Autodesk Inventor part; units mm, degrees
ref_plane "YZ Plane" through (0, 0, 0) normal (1, 0, 0) x (0, 1, 0)
ref_plane "XZ Plane" through (0, 0, 0) normal (0, 1, 0) x (-1, 0, 0)
ref_plane "XY Plane" through (0, 0, 0) normal (0, 0, 1) x (1, 0, 0)
sketch "Sketch1" plane through (0, 0, 0) normal (0, 1, 0) x (-1, 0, 0)
  line L0 (76.2, 76.2) -> (-76.2, 76.2)
  line L1 (-76.2, 76.2) -> (-76.2, -76.2)
  line L2 (-76.2, -76.2) -> (76.2, -76.2)
  line L3 (76.2, -76.2) -> (76.2, 76.2)
  point P0 (0, 0)
  dimension "d0" = 152.4
  dimension "d1" = 152.4
  dimension "d2" = 76.2
  dimension "d3" = 76.2
extrude "Extrusion1" add sketch "Sketch1" along normal blind 12.7
sketch "Sketch4" plane through (0, 12.7, 0) normal (0, 1, 0) x (1, 0, 0)
  circle A0 centre (69.85, 69.85) radius 3.175
  circle A1 centre (69.85, -69.85) radius 3.175
  circle A2 centre (-67.31, -52.07) radius 3.175
  line L0 (76.2, 76.2) -> (-76.2, 76.2)
  line L1 (76.2, -76.2) -> (76.2, 76.2)
  line L2 (-76.2, -76.2) -> (76.2, -76.2)
  line L3 (-76.2, 76.2) -> (-76.2, -76.2)
  circle A3 centre (-67.31, 52.07) radius 3.175
  point P0 (0, 0)
  dimension "d20" = 6.35
  dimension "d21" = 6.35
  dimension "d22" = 6.35
  dimension "d23" = 6.35
  dimension "d24" = 6.35
  dimension "d25" = 6.35
  dimension "d26" = 6.35
  dimension "d27" = 24.13
  dimension "d28" = 8.89
  dimension "d32" = 6.35
  dimension "d33" = 24.13
  dimension "d34" = 8.89
extrude "Extrusion6" [suppressed]
fillet "Fillet1" [suppressed]
sketch "Sketch7" plane through (0, 12.7, 0) normal (0, 1, 0) x (1, 0, 0)
  arc A0 (-76.2, -19.8745) -> (-11.9351, -76.2) centre (52.3545, 61.976) ccw
  line L0 (76.2, 76.2) -> (-76.2, 76.2)
  line L1 (76.2, -76.2) -> (76.2, 76.2)
  line L2 (-76.2, 76.2) -> (-76.2, -76.2)
  line L3 (-76.2, -76.2) -> (76.2, -76.2)
  line L4 (-76.2, 76.2) -> (-76.2, -76.2)
  arc A1 (-11.9351, -76.2) -> (-76.2, -19.8745) centre (52.3545, 61.976) ccw
  point P0 (0, 0)
  point P1 (76.2, -60.325)
  point P2 (73.025, -60.325)
  point P3 (73.025, 63.5)
  point P4 (73.025, 60.325)
  point P5 (-73.025, 63.5)
  point P6 (76.2, 60.325)
  point P7 (73.025, -63.5)
  point P8 (-76.2, 60.325)
  point P9 (-74.6455, -22.2663)
  dimension "d46" = 304.8
  dimension "d47" = 14.224
  dimension "d48" = 23.8455
sketch "Sketch8" plane through (0, 12.7, 0) normal (0, 1, 0) x (1, 0, 0)
  circle A0 centre (-38.0726, -33.782) radius 1.4224
  circle A1 centre (-44.8036, -27.051) radius 1.4224
  circle A2 centre (-51.5346, -33.782) radius 1.4224
  circle A3 centre (-51.5346, 67.818) radius 1.4224
  circle A4 centre (-44.8036, 61.087) radius 1.4224
  circle A5 centre (-38.0726, 67.818) radius 1.4224
  circle A6 centre (-53.876, 3.1912) radius 1.4224
  circle A7 centre (-53.876, 3.1912) radius 1.4224
  circle A8 centre (-44.856, 3.1912) radius 1.4224
  line L0 (-40.346, 0.6734) -> (-58.386, 0.6734)
  line L1 (-40.346, 5.7089) -> (-40.346, 0.6734)
  line L2 (-40.346, 5.7089) -> (-58.386, 5.7089)
  line L3 (-58.386, 0.6734) -> (-58.386, 5.7089)
  circle A9 centre (-53.876, 31.1756) radius 1.4224
  circle A10 centre (-44.856, 31.1756) radius 1.4224
  line L4 (-40.346, 28.6579) -> (-58.386, 28.6579)
  line L5 (-40.346, 33.6934) -> (-40.346, 28.6579)
  line L6 (-40.346, 33.6934) -> (-58.386, 33.6934)
  line L7 (-58.386, 28.6579) -> (-58.386, 33.6934)
  circle A11 centre (2.54, -39.6875) radius 3.175 construction
  circle A12 centre (2.54, 12.7127) radius 3.175 construction
  circle A13 centre (2.54, 65.1129) radius 3.175 construction
  circle A14 centre (68.58, 65.1129) radius 3.175 construction
  circle A15 centre (68.58, 12.7127) radius 3.175 construction
  circle A16 centre (68.58, -39.6875) radius 3.175 construction
extrude "Extrusion9" cut sketch "Sketch8" against normal through all contours A0 | A1 | A2 | A3 | A4 | A5 | A6 | A8 | A9 | A10
extrude "Extrusion11" cut sketch "Sketch7" against normal through all contours A0 L3 L2
sketch "Sketch10" plane through (0, 12.7, 0) normal (0, 1, 0) x (1, 0, 0)
  circle A0 centre (68.961, 72.39) radius 1.4732
  arc A1 (-76.2, -19.8745) -> (-11.9351, -76.2) centre (52.3545, 61.976) ccw
  line L0 (-11.9351, -76.2) -> (76.2, -76.2)
  line L1 (76.2, -76.2) -> (76.2, 76.2)
  line L2 (76.2, 76.2) -> (-76.2, 76.2)
  line L3 (-76.2, 76.2) -> (-76.2, -19.8745)
  circle A2 centre (-53.876, 31.1756) radius 1.4224
  circle A3 centre (-53.876, 3.1912) radius 1.4224
  circle A4 centre (-44.8036, 61.087) radius 1.4224
  circle A5 centre (-51.5346, -33.782) radius 1.4224
  circle A6 centre (-38.0726, -33.782) radius 1.4224
  circle A7 centre (-44.8036, -27.051) radius 1.4224
  circle A8 centre (-51.5346, 67.818) radius 1.4224
  circle A9 centre (-38.0726, 67.818) radius 1.4224
  circle A10 centre (-44.856, 3.1912) radius 1.4224
  circle A11 centre (-44.856, 31.1756) radius 1.4224
  circle A12 centre (40.005, 72.39) radius 1.4732
  circle A13 centre (54.483, 72.39) radius 1.4732
  circle A14 centre (25.527, 72.39) radius 1.4732
  circle A15 centre (11.049, 72.39) radius 1.4732
  circle A16 centre (68.961, -68.58) radius 1.4732
  circle A17 centre (54.483, -68.58) radius 1.4732
  circle A18 centre (40.005, -68.58) radius 1.4732
  circle A19 centre (25.527, -68.58) radius 1.4732
  circle A20 centre (11.049, -68.58) radius 1.4732
  point P0 (0, 0)
extrude "Extrusion13" cut sketch "Sketch10" against normal through all contours A0 | A12 | A13 | A14 | A15 | A16 | A17 | A18 | A19 | A20
sketch "Sketch11" plane through (0, 12.7, 0) normal (0, 1, 0) x (1, 0, 0)
  circle A0 centre (25.527, 72.39) radius 1.4732
  circle A1 centre (54.483, 72.39) radius 1.4732
  circle A2 centre (68.961, -68.58) radius 1.4732
  circle A3 centre (40.005, -68.58) radius 1.4732
  circle A4 centre (11.049, -68.58) radius 1.4732
  circle A5 centre (7.62, -42.545) radius 1.4732
  circle A6 centre (7.62, -12.9117) radius 1.4732
  circle A7 centre (7.62, 16.7217) radius 1.4732
  circle A8 centre (7.62, 46.355) radius 1.4732
  circle A9 centre (72.39, 61.1717) radius 1.4732
  circle A10 centre (72.39, 31.5383) radius 1.4732
  circle A11 centre (72.39, 1.905) radius 1.4732
  circle A12 centre (72.39, -27.7283) radius 1.4732
  circle A13 centre (72.39, -57.3617) radius 1.4732
  circle A14 centre (72.39, -42.545) radius 1.4732
  circle A15 centre (72.39, -12.9117) radius 1.4732
  circle A16 centre (72.39, 16.7217) radius 1.4732
  circle A17 centre (72.39, 46.355) radius 1.4732
  circle A18 centre (7.62, 61.1717) radius 1.4732
  circle A19 centre (7.62, 31.5383) radius 1.4732
  circle A20 centre (7.62, 1.905) radius 1.4732
  circle A21 centre (7.62, -27.7283) radius 1.4732
  circle A22 centre (7.62, -57.3617) radius 1.4732
  circle A23 centre (25.527, -68.58) radius 1.4732
  circle A24 centre (54.483, -68.58) radius 1.4732
  circle A25 centre (68.961, 72.39) radius 1.4732
  circle A26 centre (40.005, 72.39) radius 1.4732
  circle A27 centre (11.049, 72.39) radius 1.4732
  line L0 (6.985, -72.39) -> (73.025, -72.39)
  line L1 (76.2, -69.215) -> (76.2, 73.025)
  line L2 (73.025, 76.2) -> (6.985, 76.2)
  line L3 (3.81, 73.025) -> (3.81, -69.215)
  arc A28 (65.405, 62.23) -> (62.23, 65.405) centre (62.23, 62.23) ccw
  line L4 (65.405, -58.42) -> (65.405, 62.23)
  arc A29 (62.23, -61.595) -> (65.405, -58.42) centre (62.23, -58.42) ccw
  line L5 (17.78, -61.595) -> (62.23, -61.595)
  arc A30 (14.605, -58.42) -> (17.78, -61.595) centre (17.78, -58.42) ccw
  line L6 (14.605, 62.23) -> (14.605, -58.42)
  arc A31 (17.78, 65.405) -> (14.605, 62.23) centre (17.78, 62.23) ccw
  line L7 (62.23, 65.405) -> (17.78, 65.405)
  arc A32 (76.2, 73.025) -> (73.025, 76.2) centre (73.025, 73.025) ccw
  arc A33 (6.985, 76.2) -> (3.81, 73.025) centre (6.985, 73.025) ccw
  arc A34 (3.81, -69.215) -> (6.985, -72.39) centre (6.985, -69.215) ccw
  arc A35 (73.025, -72.39) -> (76.2, -69.215) centre (73.025, -69.215) ccw
  point P0 (0, 0)
extrude "Extrusion14" cut sketch "Sketch11" against normal through all contours A5 | A6 | A7 | A8 | A9 | A10 | A11 | A12 | A13 | A14 | A15 | A16 | A17 | A18 | A19 | A20 | A21 | A22 | A25
sketch "Sketch12" plane through (0, 12.7, 0) normal (0, 1, 0) x (1, 0, 0)
  line L0 (-76.2, 76.2) -> (-76.2, -19.8745)
  line L1 (76.2, 76.2) -> (-76.2, 76.2)
  circle A0 centre (-53.876, 31.1756) radius 1.4224
  circle A1 centre (-53.876, 3.1912) radius 1.4224
  line L2 (-53.876, 17.1834) -> (-44.4208, 17.1834) construction
  point P0 (0, 0)
  point P1 (-60.325, -13.9316)
  point P2 (-60.325, 48.2984)
  dimension "d63" = 15.875
  dimension "d64" = 15.875
  dimension "d75" = 13.9922
  dimension "d76" = 27.9845
  dimension "d77" = 31.115
  dimension "d78" = 31.115
hole "Hole1" at (-60.325, 12.7, 13.9316) at (-60.325, 12.7, -48.2984) direction (0, -1, 0) diameter 5.588 depth 25.4 tip angle 118
sketch "Sketch14" plane through (0, 0, 0) normal (0, -1, 0) x (1, 0, 0)
  line L0 (76.2, -76.2) -> (-76.2, -76.2)
  line L1 (-11.9351, 76.2) -> (76.2, 76.2)
  circle A0 centre (11.049, -72.39) radius 1.4732
  circle A1 centre (-38.0726, -67.818) radius 1.4224
  point P0 (0, 0)
  point P1 (-13.5118, 38.1)
  point P2 (-13.5118, -38.1)
  dimension "d79" = 38.1
  dimension "d80" = 152.4
  dimension "d81" = 38.1
  dimension "d82" = 49.1217
  dimension "d83" = 24.5608
  dimension "d84" = 24.5608
hole "Hole2" at (-13.5118, 0, 38.1) at (-13.5118, 0, -38.1) direction (0, 1, 0) diameter 6.35 depth 25.4 tip angle 118
sketch "Sketch15" plane through (0, 0, 0) normal (0, -1, 0) x (1, 0, 0)
  circle A0 centre (-13.5118, 38.1) radius 3.175
  circle A1 centre (-13.5118, -38.1) radius 3.175
  circle A2 centre (72.39, -31.5383) radius 1.4732
  circle A3 centre (7.62, -31.5383) radius 1.4732
  circle A4 centre (7.62, 42.545) radius 1.4732
  point P0 (0, 0)
  point P1 (40.005, -38.1)
  point P2 (40.005, 38.1)
  dimension "d92" = 38.1
  dimension "d93" = 38.1
  dimension "d94" = 38.1
  dimension "d95" = 38.1
  dimension "d96" = 64.77
  dimension "d97" = 32.385
  dimension "d98" = 32.385
hole "Hole3" at (40.005, 0, -38.1) at (40.005, 0, 38.1) direction (0, 1, 0) diameter 6.35 depth 9.525
thread "Thread1"
thread "Thread2"
thread "Thread3"
thread "Thread4"
thread "Thread5"
thread "Thread6"
thread "Thread7"
thread "Thread8"
thread "Thread9"
thread "Thread10"
thread "Thread11"
thread "Thread12"
thread "Thread13"
thread "Thread14"
thread "Thread15"
thread "Thread16"
thread "Thread17"
thread "Thread18"
thread "Thread19"
thread "Thread20"
thread "Thread21"
thread "Thread22"
thread "Thread23"
thread "Thread24"
thread "Thread25"
thread "Thread26"
thread "Thread27"
thread "Thread28"
thread "Thread29"
thread "Thread30"
thread "Thread31"
thread "Thread32"
thread "Thread33"
thread "Thread34"
thread "Thread35"
thread "Thread36"
thread "Thread37"
thread "Thread38"
thread "Thread39"
thread "Thread40"
thread "Thread41"
thread "Thread42"
thread "Thread43"
thread "Thread44"
thread "Thread45"
sketch "Sketch16" plane through (0, 0, 0) normal (0, -1, 0) x (1, 0, 0)
  line L0 (76.2, 76.2) -> (76.2, -76.2)
  line L1 (76.2, -76.2) -> (-76.2, -76.2)
  line L2 (76.2, 76.2) -> (69.85, 76.2)
  line L3 (69.85, 76.2) -> (69.85, -76.2)
  line L4 (69.85, -76.2) -> (76.2, -76.2)
  line L5 (76.2, -76.2) -> (76.2, 76.2)
  point P0 (0, 0)
  dimension "d196" = 6.35
extrude "Extrusion15" cut sketch "Sketch16" against normal blind 6.35
equation "\"d21\" = d20"
equation "\"d22\" = d20"
equation "\"d24\" = d23"
equation "\"d25\" = d24"
equation "\"d26\" = d23"
equation "\"d32\" = d20"
equation "\"d33\" = d27"
equation "\"d34\" = d28"
equation "\"d75\" = 0.5 * d76"
properties part number "Base Plate Mk 3" material "Aluminum 6061"
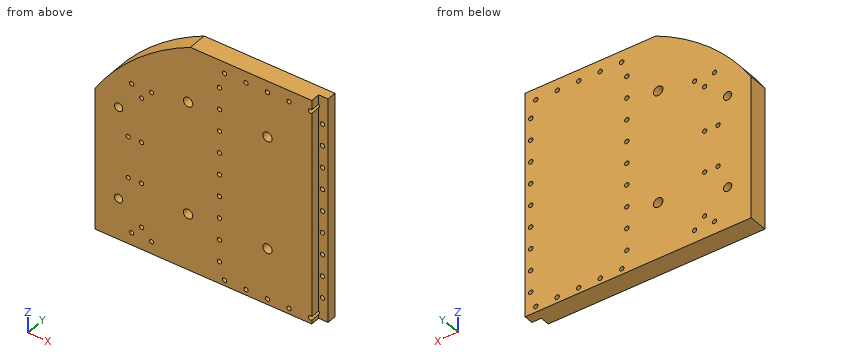
Check sheet for the modelled part. Datum: model origin and axes. Units: mm. Round coordinates to 2 decimals unless told otherwise and drop trailing zeros. Write each loop counter-clockwise with the first axis right and the second up, starting at its lowest first coordinate (ties: lowest second). Pieces come first, ordered by that corner, then holes. Notation, with made-up numbers: (54.25, -19.5) -> (104.25, -19.5) arc R28 ccw to (104.25, 14.5) -> close; hole circle Ø6 at (-3, 20.5). An arc over 180 degrees is marked (long way). One line per question, with ' | ' between items. Start each with the question number.
1. Sectioned sample at A-A, the plane z = -38.1. Record the cut outline in (x, y) (3 decimals).
2. Sectioned sample at C-C, the plane x = -34. Record the cut outline in (y, z), then the cut area to 3 significant figures.
3. Depth check by flat-ended pin: pin 1 (2.5 mm diameter, centred on x = -53.88, z = -31.18, fed in from -Y); pin 2 (3.5 mm diameter, centred on x = -44.8, z = 27.05, fed in from +Y); pin 3 (4.5 mm diameter, centred on x = 72.39, z = 57.36, fed in from -Y); pin 4 (7 mm diameter, centred on y = 2.5, z = 73.5, fed in from +X). Enter the tip coordinate at first touch or a pass-through.
4. Scan lines: line 1 along X through (y, z) = (6.75, -72.39); line 2 along Z through (x, y) = (26.5, 2.25); line 3 along Z through (x, y) = (-62.5, 1.5). Record each from-to range of solid material in increasing order. Write a range as from..to.
5. Sectioned sample at B-B, the plane y = 1.75. Count the separate pieces of the cut face and the enclosed holes in it, then the cut area to 3 significant figures.
Taken from the geometry:
1) outline: (-76.2, 0) -> (-16.687, 0) -> (-16.687, 12.7) -> (-76.2, 12.7) -> close; (-10.337, 0) -> (36.83, 0) -> (36.83, 9.525) -> (43.18, 9.525) -> (43.18, 0) -> (69.85, 0) -> (69.85, 6.35) -> (76.2, 6.35) -> (76.2, 12.7) -> (-10.337, 12.7) -> close
2) outline: (0, -76.2) -> (12.7, -76.2) -> (12.7, 63.6) -> (0, 63.6) -> close | area: 1,780 mm^2
3) pin 1: passes through | pin 2: stops at y = 12.7 | pin 3: stops at y = 6.35 | pin 4: stops at x = 69.85
4) line 1: x = -76.2..9.58, 12.52..24.05, 27..38.53, 41.48..53.01, 55.96..67.49, 70.43..76.2 | line 2: z = -76.2..-73.5, -71.28..67.47, 69.69..76.2 | line 3: z = -76.2..-50.05, -46.54..12.18, 15.69..38.19
5) separate pieces: 1 | enclosed holes: 33 | area: 20,400 mm^2
